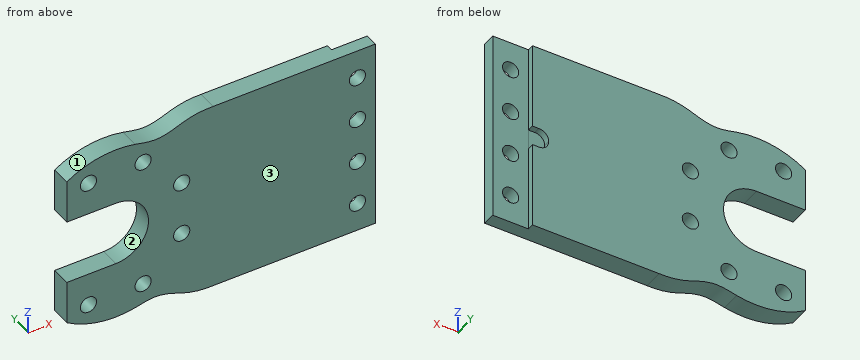
Autodesk Inventor part; units mm, degrees
ref_plane "Work Plane1" through (45, 0, 15) normal (1, 0, 0) x (0, 0, -1)
ref_plane "YZ Plane" through (0, 0, 0) normal (1, 0, 0) x (0, 1, 0)
ref_plane "XZ Plane" through (0, 0, 0) normal (0, 1, 0) x (-1, 0, 0)
sketch "Sketch1" plane through (0, 0, 0) normal (0, 1, 0) x (-1, 0, 0)
  line L0 (-40, 15) -> (0, 15) construction
  line L1 (15, 15) -> (15, -15) construction
  line L2 (15, -15) -> (0, -15) construction
  line L3 (-40, -15) -> (-40, 15)
  line L4 (15, 0) -> (-40, 0) construction
  line L5 (-28.4, 0) -> (23.4, 0) construction
  circle A0 centre (0, 0) radius 11 construction
  line L6 (11, 15) -> (11, -15) construction
  circle A1 centre (0, 0) radius 5.05 construction
  line L7 (0, 5.05) -> (7.55, 5.05) construction
  line L8 (0, -5.05) -> (7.55, -5.05) construction
  line L9 (15, 15) -> (15, 5) construction
  line L10 (15, -5) -> (15, -15) construction
  arc A2 (0, 5.05) -> (0, -5.05) centre (0, 0) ccw
  circle A3 centre (0, 0) radius 15 construction
  arc A4 (0, -15) -> (14.1421, -5) centre (0, 0) ccw construction
  arc A5 (14.1421, 5) -> (0, 15) centre (0, 0) ccw construction
  line L11 (0, -15) -> (-40, -15) construction
  line L12 (0, 15) -> (15, 15) construction
  arc A6 (11, -8.6603) -> (11, 8.6603) centre (0, 0) ccw construction
  line L13 (-3, -15) -> (-3, 15) construction
  arc A7 (-3, -13.6748) -> (7.55, -11.7897) centre (0, 0) ccw
  line L14 (7.55, 5.05) -> (0, 5.05)
  line L15 (-15, -18.6523) -> (-15, 18.2394) construction
  line L16 (-40, -15) -> (-15, -15)
  line L17 (-40, 15) -> (-15, 15)
  spline S0 degree 4 poles (-3, -13.6748) (-4.5129, -13.3429) (-7.4407, -12.2328) (-10.459, -15) (-13.4863, -15) (-15, -15) knots 0 0 0 0 0 0.5 1 1 1 1 1
  spline S1 degree 4 poles (-3, 13.6748) (-4.5129, 13.3429) (-7.4407, 12.2328) (-10.459, 15) (-13.4863, 15) (-15, 15) knots 0 0 0 0 0 0.5 1 1 1 1 1
  line L18 (5.05, -15) -> (5.05, 15) construction
  line L19 (7.55, -11.7897) -> (7.55, -5.05)
  line L20 (7.55, 5.05) -> (7.55, 11.7897)
  line L21 (7.55, -5.05) -> (11, -5.05) construction
  line L22 (7.55, 5.05) -> (9.7723, 5.05) construction
  arc A8 (7.55, 11.7897) -> (7.55, -11.7897) centre (0, 0) ccw construction
  arc A9 (7.55, 11.7897) -> (-3, 13.6748) centre (0, 0) ccw
  line L23 (0, -5.05) -> (7.55, -5.05)
  line L24 (0, -26.0306) -> (0, 25.6178) construction
  line L25 (35.28, 0) -> (-47.88, 0) construction
  point P0 (13.0767, -5)
  dimension "d1" = 22
  dimension "d0" = 30
  dimension "d2" = 40
  dimension "d3" = 10.1
  dimension "d4" = 30
  dimension "d5" = 28
  dimension "d6" = 15
  dimension "d7" = 12
  dimension "d8" = 2.5
extrude "Extrusion1" add sketch "Sketch1" along normal blind 3
sketch "Sketch2" plane through (0, 3, 0) normal (0, 1, 0) x (1, 0, 0)
  circle A0 centre (0, 0) radius 11 construction
  line L0 (-21.2, 0) -> (50.2, 0) construction
  line L1 (0, 21) -> (0, -21) construction
  line L2 (0, 0) -> (-4.2095, -10.1627) construction
  point P0 (-4.2095, -10.1627)
  point P1 (4.2095, -10.1627)
  point P2 (10.1627, -4.2095)
  point P3 (10.1627, 4.2095)
  point P4 (4.2095, 10.1627)
  point P5 (-4.2095, 10.1627)
  dimension "d19" = 22
  dimension "d20" = 225
  dimension "d68" = 22.5
hole "Hole1" at (-4.2095, 3, 10.1627) at (-4.2095, 3, -10.1627) at (4.2095, 3, -10.1627) at (10.1627, 3, -4.2095) at (10.1627, 3, 4.2095) at (4.2095, 3, 10.1627) direction (0, -1, 0) diameter 2.5 end through all
sketch "Sketch3" plane through (0, 3, 0) normal (0, 1, 0) x (1, 0, 0)
  circle A0 centre (-4.2095, -10.1627) radius 1.25 construction
  circle A1 centre (4.2095, -10.1627) radius 1.25 construction
  circle A2 centre (10.1627, -4.2095) radius 1.25 construction
  circle A3 centre (10.1627, 4.2095) radius 1.25 construction
  circle A4 centre (4.2095, 10.1627) radius 1.25 construction
  circle A5 centre (-4.2095, 10.1627) radius 1.25 construction
  point P0 (0, 0)
sketch "Sketch4" plane through (0, 3, 0) normal (0, 1, 0) x (1, 0, 0)
  line L0 (37, -21.9283) -> (37, 20.7608) construction
  line L1 (40, -15) -> (40, 15) construction
  line L2 (15, -15) -> (40, -15) construction
  point P0 (0, 0)
  point P1 (37, -10.5)
  point P2 (37, -3.5)
  point P3 (37, 3.5)
  point P4 (37, 10.5)
  dimension "d29" = 3
  dimension "d30" = 4.5
  dimension "d33" = 7
hole "Hole2" [suppressed]
sketch "Sketch6" plane through (0, 3, 0) normal (0, 1, 0) x (1, 0, 0)
  line L0 (15, -15) -> (40, -15)
  line L1 (40, -15) -> (34.5, -15)
  line L2 (34.5, -15) -> (34.5, 15)
  line L3 (34.5, 15) -> (40, 15)
  line L4 (40, 15) -> (40, -15)
  line L5 (37.25, 15) -> (37.25, -15) construction
  point P0 (0, 0)
  point P1 (37.25, -10.5)
  point P2 (37.25, -3.5)
  point P3 (37.25, 3.5)
  point P4 (37.25, 10.5)
  dimension "d47" = 5.5
  dimension "d55" = 30
  dimension "d56" = 7
  dimension "d57" = 7
  dimension "d58" = 7
  dimension "d59" = 4.5
  dimension "d60" = 4.5
extrude "Extrusion2" cut sketch "Sketch6" against normal blind 1
sketch "Sketch7" plane through (0, 3, 0) normal (0, 1, 0) x (1, 0, 0)
  line L0 (34.5, -15) -> (34.5, 15)
  line L1 (34.5, 15) -> (15, 15)
  arc A0 (3, 13.6748) -> (-7.55, 11.7897) centre (0, 0) ccw
  line L2 (-7.55, 11.7897) -> (-7.55, 5.05)
  line L3 (-7.55, 5.05) -> (0, 5.05)
  arc A1 (0, -5.05) -> (0, 5.05) centre (0, 0) ccw
  line L4 (0, -5.05) -> (-7.55, -5.05)
  line L5 (-7.55, -5.05) -> (-7.55, -11.7897)
  arc A2 (-7.55, -11.7897) -> (3, -13.6748) centre (0, 0) ccw
  line L6 (15, -15) -> (34.5, -15)
  circle A3 centre (10.1627, -4.2095) radius 1.25
  circle A4 centre (4.2095, 10.1627) radius 1.25
  circle A5 centre (-4.2095, -10.1627) radius 1.25
  circle A6 centre (-4.2095, 10.1627) radius 1.25
  circle A7 centre (10.1627, 4.2095) radius 1.25
  circle A8 centre (4.2095, -10.1627) radius 1.25
  line L7 (34.5, 1.55) -> (32, 1.55)
  line L8 (32, 1.55) -> (32, -1.55)
  line L9 (32, -1.55) -> (34.5, -1.55)
  line L10 (34.5, 0) -> (32, 0) construction
  point P0 (0, 0)
  dimension "d50" = 3.1
  dimension "d51" = 2.5
extrude "Extrusion3" cut sketch "Sketch7" against normal blind 1 contours L9 L8 L7 L0
fillet "Fillet1" radius 1.5 2 edges at (32, 2.5, 1.55) (32, 2.5, -1.55)
hole "Hole3" at (37.25, 3, -10.5) at (37.25, 3, -3.5) at (37.25, 3, 3.5) at (37.25, 3, 10.5) direction (0, -1, 0) diameter 2.5 end through all
ref_plane "Work Plane1" through (45, 0, 15) normal (1, 0, 0) x (0, 0, -1)
equation "\"d3\" = horn_radius_clearance"
equation "\"d19\" = d21"
equation "\"d47\" = base_border_height"
equation "\"d9\" = 30"
equation "\"d10\" = 22"
equation "\"horn_radius_clearance\" = 10.1"
equation "\"d14\" = 2 * d13"
equation "\"d21\" = 22"
equation "\"base_2_axis\" = 40"
equation "\"base_border_height\" = 5.5"
properties part number "test_side_u64" material "Aluminum 6061"
Design review of the part built by this model. Coordinates are the model's own, in mm. Face numbers are marked on the shaded views. Coordinates: 2 decimals unless noted, no trailing zeros. Order: outer loops, then holes, each group sorted by start corner. A loop starts at its lowest first (then second) coordinate and runs counter-clockwise, first axis right, second up. Notation, with made-up numbers: M -9,2.25 L 0,2.25 A27 ccw 0,41.25 Z; hole C -10,20.25 d6. An arc over 180 degrees is marked long. Answer as a JSON object with one key per item and string values. Group by question number.
1) For pin 1 (0.9 mm diameter, centred on x = -5, y = 1, fed in from -Z); pin 2 (3 mm diameter, centred on x = 38, z = -4, fed in from +Y); pin 3 (0.8 mm diameter, centred on y = 2.5, z = -6, fed in from +X), all flat-tipped, find the tip position at first contact; note any pin that passes through.
2) Add section A-A, the plane x = 37.25. Write out the cut boundary in (y, z), then the cut area to 3 significant figures.
3) Add section D-D, the plane z = -10.5. Write out the cut boundary in (x, y), then the cut area to 3 significant figures.
4) Add section C-C, the plane x = -2.5. Write out the cut boundary in (y, z).
5) Mouldability with a two-part tool opening along Z and no side actions: class the marked faces 1, 2 and 3 as pulls with the +Z half, pulls with the -Z half, needs draft (parallel to the pull), parting line crosses it, or undercut.
6) Add section B-B, the plane z = -3.5. Write out the cut boundary in (x, y), then the cut area to 3 significant figures.
7) Wall thickness on L1, parallel to Z at x = 37.25, y = 0.95; L2, parallel to X at y = 2.25, z = 10.5; L3, parallel to X at y = 0.95, z = -3.5: over which ranges is each line inside the solid? List them lowest first.
Computed values:
{
 "1": {"pin 1": "stops at z = -13.24", "pin 2": "stops at y = 2", "pin 3": "stops at x = 34.5"},
 "2": {"outline": "M 0,-15 L 2,-15 L 2,-11.75 L 0,-11.75 Z; M 0,-9.25 L 2,-9.25 L 2,-4.75 L 0,-4.75 Z; M 0,-2.25 L 2,-2.25 L 2,2.25 L 0,2.25 Z; M 0,4.75 L 2,4.75 L 2,9.25 L 0,9.25 Z; M 0,11.75 L 2,11.75 L 2,15 L 0,15 Z", "area": "40.0 mm^2"},
 "3": {"outline": "M -7.55,0 L -5.41,0 L -5.41,3 L -7.55,3 Z; M -3.01,0 L 3.01,0 L 3.01,3 L -3.01,3 Z; M 5.41,0 L 36,0 L 36,2 L 34.5,2 L 34.5,3 L 5.41,3 Z; M 38.5,0 L 40,0 L 40,2 L 38.5,2 Z", "area": "118 mm^2"},
 "4": {"outline": "M 0,-13.77 L 3,-13.77 L 3,-5.05 L 0,-5.05 Z; M 0,5.05 L 3,5.05 L 3,13.77 L 0,13.77 Z"},
 "5": {"face 1": "pulls with the +Z half", "face 2": "undercut", "face 3": "needs draft"},
 "6": {"outline": "M 3.64,0 L 9.13,0 L 9.13,3 L 3.64,3 Z; M 11.19,0 L 36,0 L 36,2 L 34.5,2 L 34.5,3 L 11.19,3 Z; M 38.5,0 L 40,0 L 40,2 L 38.5,2 Z", "area": "92.4 mm^2"},
 "7": {"L1": "z = -15 to -11.75, -9.25 to -4.75, -2.25 to 2.25, 4.75 to 9.25, 11.75 to 15", "L2": "x = -7.55 to -5.41, -3.01 to 3.01, 5.41 to 34.5", "L3": "x = 3.64 to 9.13, 11.19 to 36, 38.5 to 40"}
}
